```python
from build123d import *

# Parameters (mm, degrees)
SKETCH_1_R      = 2
EXTRUDE_1_DEPTH = 1.5
SKETCH_2_R      = 1.5
EXTRUDE_2_DEPTH = 20
SKETCH_3_R      = 6
EXTRUDE_3_DEPTH = 2


with BuildPart() as part:
    # 草图1 → 凸台-拉伸1 (new, symmetric)
    with BuildSketch(Plane.XY):
        with BuildLine():
            Line((0, 0), (6, 0))
            Line((6, 0), (6, 10))
            ThreePointArc((6, 10), (3, 13), (0, 10))
            Line((0, 10), (0, 0))
        make_face()
        with Locations((3, 10)):
            Circle(SKETCH_1_R, mode=Mode.SUBTRACT)
    extrude(amount=EXTRUDE_1_DEPTH, both=True)

    # 草图2 → 凸台-拉伸2 (add)
    with BuildSketch(Plane.XZ):
        with Locations(Location((3, 0, 0), (0, 0, 270))):
            Circle(SKETCH_2_R)
    extrude(amount=EXTRUDE_2_DEPTH)

    # 草图3 → 凸台-拉伸3 (add)
    with BuildSketch(Plane.XZ.offset(20)):
        with Locations(Location((3, 0, 0), (0, 0, 270))):
            Circle(SKETCH_3_R)
    extrude(amount=EXTRUDE_3_DEPTH)


solid = part.part
```
Can you work these out from the model? Positions are in its coordinate system, mm. A direction names the side the tool comes from. Coordinates: 2 decimals unless noted, no trailing zeros. Loops run counter-clockwise (first coordinate to the right, second up) from the corner with the lowest first, then second, coordinate; pieces in that order, holes last. Notation, with made-up numbers: M 32,-10 L 43,-10 A20 ccw 43,-4 Z; hole C -24.5,30 d10. An arc over 180 degrees is marked long. Put each result on its own line as item: value. Start each with the question number.
(1) Which directions (+Z, -Z, +X, -X, +Y, -Y) give clear straight access to the entire face, cutting with the end or side of a thin tool? Please do faces 1 (the face through (3, 5, 1.5)), 2 (the face through (1.8, -20, -1.2)), 3 (the face through (5, 0, 0)), 4 (the face through (0, 5, 0)).
(2) Imagine slicing it at B-B on x = 0.5. List the corners of the cut face in (y, z) for me, and give its area (3 significant figures).
(3) Imagine slicing it at D-D on z = -3.5. List the corners of the cut face in (x, y) for me.
(4) Imagine slicing it at A-A on z = 0. List the corners of the cut face in (x, y) for me.
(5) Will these pins go through, and if not, where does the flat tip stop? pin 1 Ø3 at (y, z) = (-11, 0.5) entering from -X; pin 2 Ø1.5 at (y, z) = (3.5, 0.5) entering from -X; pin 3 Ø1.8 at (x, y) = (3, 7) entering from +Z.
(6) Imagine slicing it at C-C on y = 4. List the corners of the cut face in (x, z) for me.
(7) I need wall thicknesses on probe 1 along Y at (x, z) = (3, -0.4); probe 2 along X at (y, z) = (7.5, 0.25); probe 3 along Y at (x, z) = (1.5, -4.5). Which ranges of each line are inside material? Lowest first, please.
(8) We'd pull the mould along Y, two halves only. Please class faces 5 (the face through (3, 13, 0)), 6 (the face through (4.802, -20.986, -5.723)), 7 (the face through (1, 0, 0)): +Y half, -Y half, draft (parallel to the pull), parting line (faces both ways), or undercut.
Worked answers:
1. face 1: +Z, +X, -X, +Y
1. face 2: none
1. face 3: +X
1. face 4: +Z, -Z, -X, +Y
2. outline: M -22,-5.45 L -20,-5.45 L -20,5.45 L -22,5.45 Z; M 0,-1.5 L 11.66,-1.5 L 11.66,1.5 L 0,1.5 Z
2. area: 56.8 mm2
3. outline: M -1.87,-22 L 7.87,-22 L 7.87,-20 L -1.87,-20 Z
4. outline: M -3,-22 L 9,-22 L 9,-20 L 4.5,-20 L 4.5,0 L 6,0 L 6,10 A3 ccw 0,10 L 0,0 L 1.5,0 L 1.5,-20 L -3,-20 Z; hole C 3,10 d4
5. pin 1: stops at x = 1.5
5. pin 2: stops at x = 0
5. pin 3: stops at z = 1.5
6. outline: M 0,-1.5 L 6,-1.5 L 6,1.5 L 0,1.5 Z
7. probe 1: y = -22 to 8, 12 to 13
7. probe 2: x = 0 to 6
7. probe 3: y = -22 to -20
8. face 5: +Y half
8. face 6: draft
8. face 7: undercut
